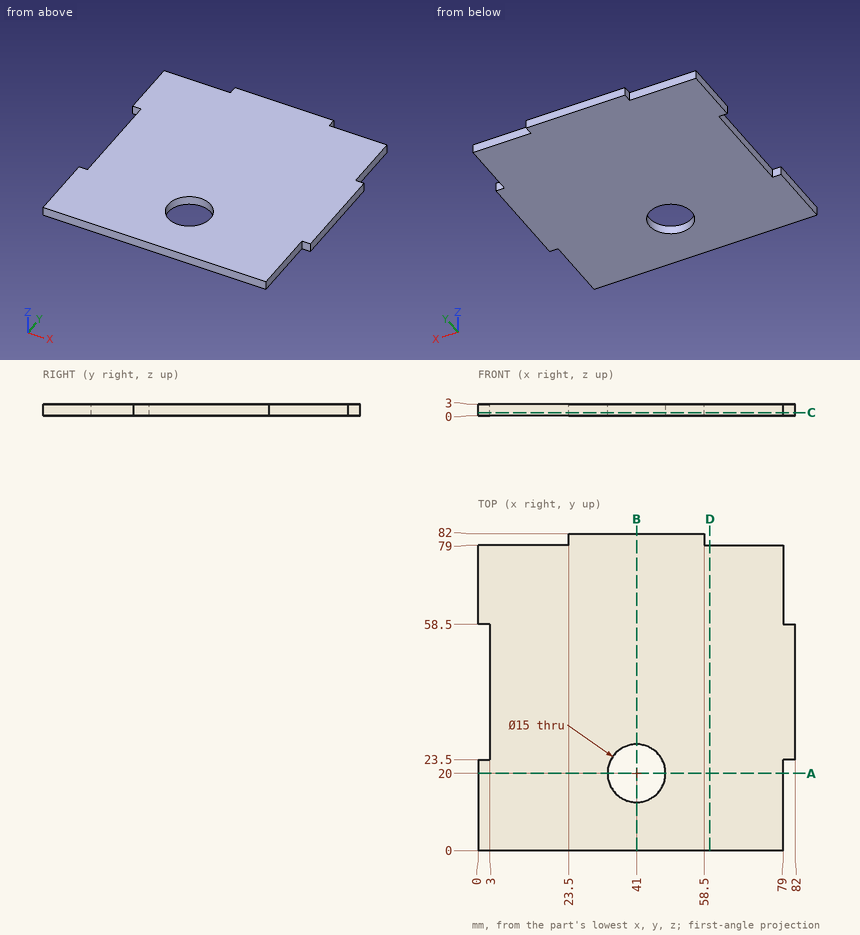
Could you check a few things on this drawing? It's one solid part, dimensions in mm from its lowest x, y, z. Give positions to 0.01 mm unless a question says otherwise; leave off trailing zeros. Order: outer loops, then holes, each group sorted by start corner. A loop starts at its lowest first (then second) coordinate and runs counter-clockwise, first axis right, second up. Notation, with made-up numbers: (10, -34.5) - (34, -34.5) arc R21 ccw to (34, -9.5) - close; hole circle Ø3 at (-33.5, 23.5). An arc over 180 degrees is marked (long way). Answer as a JSON object with one key per item and string values. Group by question number.
Item 1: For P1, Ø1.5, axis at y = 73.5, z = 1, coming from the +X side; P2, Ø1.5, axis at y = 80, z = 1.5, coming from the -X side; P3, Ø1.5, axis at x = 14.5, z = 1.5, coming from the +Y side, each with a flat end and sliding along its axis, tell me the tip position at first contact or that it passes through.
Item 2: If we section it at C-C on z = 0.8: Please give me the cut outline in (x, y).
Item 3: Please list where these lines run through material, in increasing order: probe 1 along Y at (x, z) = (41, 0.9); probe 2 along Y at (x, z) = (73, 0.15).
Item 4: If we section it at B-B on x = 41: Please give me the cut outline in (y, z), and give its area (3 significant figures).
Item 5: If we section it at D-D on x = 60: Please give me the cut outline in (y, z).
Item 6: If we section it at A-A on y = 20: Please give me the cut outline in (x, z), and give its area (3 significant figures).
Result set:
{
 "1": {"P1": "x = 79", "P2": "x = 23.5", "P3": "y = 79"},
 "2": {"outline": "(0, 0) - (79, 0) - (79, 23.5) - (82, 23.5) - (82, 58.5) - (79, 58.5) - (79, 79) - (58.5, 79) - (58.5, 82) - (23.5, 82) - (23.5, 79) - (0, 79) - (0, 58.5) - (3, 58.5) - (3, 23.5) - (0, 23.5) - close; hole circle Ø15 at (41, 20)"},
 "3": {"probe 1": "0 to 12.5, 27.5 to 82", "probe 2": "0 to 79"},
 "4": {"outline": "(0, 0) - (12.5, 0) - (12.5, 3) - (0, 3) - close; (27.5, 0) - (82, 0) - (82, 3) - (27.5, 3) - close", "area": "201 mm²"},
 "5": {"outline": "(0, 0) - (79, 0) - (79, 3) - (0, 3) - close"},
 "6": {"outline": "(0, 0) - (33.5, 0) - (33.5, 3) - (0, 3) - close; (48.5, 0) - (79, 0) - (79, 3) - (48.5, 3) - close", "area": "192 mm²"}
}
